Model file for the job. Use its own axes, mm. Coordinates: 2 decimals unless noted, no trailing zeros. Loops run counter-clockwise (first coordinate to the right, second up) from the corner with the lowest first, then second, coordinate; pieces in that order, holes last. Notation, with made-up numbers: (-30.75, 24.5) -> (8.25, 24.5) arc R23 ccw to (8.25, 52.5) -> close; hole circle Ø8 at (9.5, -25.75). An arc over 180 degrees is marked (long way). Use one line per item in the form item = value.
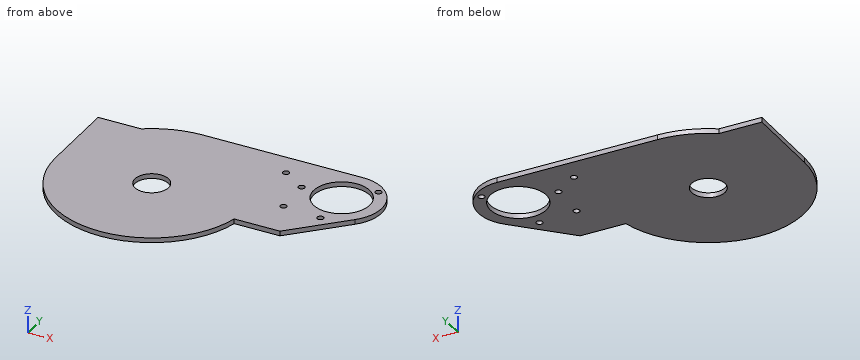
```python
from build123d import *

# Parameters (mm, degrees)
SKETCH1_R           = 10.5
SKETCH1_R_2         = 17.5
BOSS_EXTRUDE1_DEPTH = 3
CUT_EXTRUDE1_REACH  = 140.687
SKETCH2_R           = 2
CUT_EXTRUDE2_REACH  = 140.687
SKETCH3_R           = 2


with BuildPart() as part:
    # Sketch1 → Boss-Extrude1 (new body)
    # profile 1 of 2: a face of its own
    with BuildSketch(Plane.XY):
        with BuildLine():
            ThreePointArc((-60, 0), (-52.867640737, 28.372743309), (-33.166247904, 50))
            Line((-33.166247904, 50), (-60, 50))
            Line((-60, 50), (-60, 0))
        make_face()
    # profile 2 of 2: a face of its own
    with BuildSketch(Plane.XY):
        with BuildLine():
            ThreePointArc((0, 60), (-17.320508076, 57.445626465), (-33.166247904, 50))
            ThreePointArc((-33.166247904, 50), (-52.867640737, 28.372743309), (-60, 0))
            ThreePointArc((-60, 0), (-6.678621673, -59.627141576), (58.513200418, -13.274237334))
            Line((58.513200418, -13.274237334), (87.081101726, -13.274237334))
            Line((87.081101726, -13.274237334), (117.67766953, 17.32233047))
            ThreePointArc((117.67766953, 17.32233047), (123.096988313, 44.567085809), (100, 60))
            Line((100, 60), (0, 60))
        make_face()
        Circle(SKETCH1_R, mode=Mode.SUBTRACT)
        with Locations((100, 35)):
            Circle(SKETCH1_R_2, mode=Mode.SUBTRACT)
    extrude(amount=BOSS_EXTRUDE1_DEPTH)

    # Sketch2 → Cut-Extrude1 (cut, up to next)
    with BuildSketch(Plane.XY.offset(3), mode=Mode.PRIVATE) as cut_extrude1_sk1:
        with Locations((60, 45)):
            Circle(SKETCH2_R)
    cut_extrude1_tool1 = extrude(cut_extrude1_sk1.sketch, amount=-CUT_EXTRUDE1_REACH, mode=Mode.PRIVATE) & part.part
    # Sketch2 → Cut-Extrude1 (cut, up to next)
    with BuildSketch(Plane.XY.offset(3), mode=Mode.PRIVATE) as cut_extrude1_sk2:
        with Locations((76, 11.725762666)):
            Circle(SKETCH2_R)
    cut_extrude1_tool2 = extrude(cut_extrude1_sk2.sketch, amount=-CUT_EXTRUDE1_REACH, mode=Mode.PRIVATE) & part.part
    add(cut_extrude1_tool1.solids().sort_by_distance((60, 45, 3))[0], mode=Mode.SUBTRACT)
    add(cut_extrude1_tool2.solids().sort_by_distance((76, 11.725763, 3))[0], mode=Mode.SUBTRACT)

    # Sketch3 → Cut-Extrude2 (cut, up to next)
    with BuildSketch(Plane.XY.offset(3), mode=Mode.PRIVATE) as cut_extrude2_sk1:
        with Locations((100, 10)):
            Circle(SKETCH3_R)
    cut_extrude2_tool1 = extrude(cut_extrude2_sk1.sketch, amount=-CUT_EXTRUDE2_REACH, mode=Mode.PRIVATE) & part.part
    # Sketch3 → Cut-Extrude2 (cut, up to next)
    with BuildSketch(Plane.XY.offset(3), mode=Mode.PRIVATE) as cut_extrude2_sk2:
        with Locations((75, 35)):
            Circle(SKETCH3_R)
    cut_extrude2_tool2 = extrude(cut_extrude2_sk2.sketch, amount=-CUT_EXTRUDE2_REACH, mode=Mode.PRIVATE) & part.part
    # Sketch3 → Cut-Extrude2 (cut, up to next)
    with BuildSketch(Plane.XY.offset(3), mode=Mode.PRIVATE) as cut_extrude2_sk3:
        with Locations((115.0260191, 50.0260191)):
            Circle(SKETCH3_R)
    cut_extrude2_tool3 = extrude(cut_extrude2_sk3.sketch, amount=-CUT_EXTRUDE2_REACH, mode=Mode.PRIVATE) & part.part
    add(cut_extrude2_tool1.solids().sort_by_distance((100, 10, 3))[0], mode=Mode.SUBTRACT)
    add(cut_extrude2_tool2.solids().sort_by_distance((75, 35, 3))[0], mode=Mode.SUBTRACT)
    add(cut_extrude2_tool3.solids().sort_by_distance((115.026019, 50.026019, 3))[0], mode=Mode.SUBTRACT)


solid = part.part
```
Q1. Band-saw the part on B-B, the plane x = 3. Write the cut outline in (y, z), and give its area (3 significant figures).
Result:
outline = (-59.92, 0) -> (-10.06, 0) -> (-10.06, 3) -> (-59.92, 3) -> close; (10.06, 0) -> (60, 0) -> (60, 3) -> (10.06, 3) -> close
area = 299 mm2
Q2. Band-saw the part on D-D, the plane z = 0.9. Write the cut outline in (x, y), and give its area (3 significant figures).
Result:
outline = (-60, 0) arc R60 ccw to (58.51, -13.27) -> (87.08, -13.27) -> (117.68, 17.32) arc R25 ccw to (100, 60) -> (0, 60) arc R60 ccw to (-33.17, 50) -> (-60, 50) -> close; hole circle Ø21 at (0, 0); hole circle Ø4 at (60, 45); hole circle Ø4 at (75, 35); hole circle Ø4 at (76, 11.73); hole circle Ø35 at (100, 35); hole circle Ø4 at (100, 10); hole circle Ø4 at (115.03, 50.03)
area = 15,000 mm2
Q3. Band-saw the part on A-A, the plane y = 35. Write the cut outline in (x, z), and give its area (3 significant figures).
Result:
outline = (-60, 0) -> (73, 0) -> (73, 3) -> (-60, 3) -> close; (77, 0) -> (82.5, 0) -> (82.5, 3) -> (77, 3) -> close; (117.5, 0) -> (125, 0) -> (125, 3) -> (117.5, 3) -> close
area = 438 mm2
Q4. Wall check: line 1 along Y through (x, z) = (100, 2.1); line 2 along X through (y, z) = (11, 0.5); line 3 along Y through (x, z) = (0, 1.45). Give the ranges that are in metal, low to high.
Result:
line_1 = -0.36 to 8, 12 to 17.5, 52.5 to 60
line_2 = -60 to 74.14, 77.86 to 98.27, 101.73 to 111.36
line_3 = -60 to -10.5, 10.5 to 60
Q5. Pin check, flat tips, straight feed: pin 1 Ø1 at (x, z) = (-31.5, 2.5) entering from -Y; pin 2 Ø12.5 at (x, y) = (0, 0) entering from +Z; pin 3 Ø1 at (y, z) = (42, 2) entering from +X. Stop position of each tip, or through.
Result:
pin_1 = -51.37
pin_2 = through
pin_3 = 124.14
Q6. Band-saw the part on C-C, the plane y = -8. Write the cut outline in (x, z).
Result:
outline = (-59.46, 0) -> (-6.8, 0) -> (-6.8, 3) -> (-59.46, 3) -> close; (6.8, 0) -> (92.36, 0) -> (92.36, 3) -> (6.8, 3) -> close
